```python
from build123d import *

# Parameters (mm, degrees)
SKETCH_1_W                   = 60
SKETCH_1_H                   = 60
EXTRUDE_1_DEPTH              = 4
HOLE_WIZARD_M3_1_D           = 3.4
HOLE_WIZARD_M3_1_CSINK_D     = 6.6
HOLE_WIZARD_M3_1_CSINK_ANGLE = 90
HOLE_WIZARD_M4_1_AT_2_COUNT  = 2
HOLE_WIZARD_M4_1_AT_2_PITCH  = 19
HOLE_WIZARD_M4_1_AT_3_COUNT  = 2
HOLE_WIZARD_M4_1_AT_3_PITCH  = 38
HOLE_WIZARD_1_D              = 3
SKETCH_9_W                   = 12
SKETCH_9_H                   = 19
SKETCH_9_R                   = 1.5
EXTRUDE_3_DEPTH              = 4
CHAMFER_1_SIZE               = 0.5
SKETCH_10_W                  = 72
SKETCH_10_H                  = 4
EXTRUDE_4_DEPTH              = 20


with BuildPart() as part:
    # 草图1 → 凸台-拉伸1 (new body)
    with BuildSketch(Plane(origin=(0, 0, 0), x_dir=(1, 0, 0), z_dir=(0, 1, 0))):
        Rectangle(SKETCH_1_W, SKETCH_1_H)
    extrude(amount=EXTRUDE_1_DEPTH)

    # M3 十字槽沉头木螺钉的锥形沉头孔1 (through all)
    with Locations(Plane(origin=(0, 4, 0), x_dir=(1, 0, 0), z_dir=(0, 1, 0))):
        with Locations((-10, 10), (10, 10), (10, -10), (-10, -10)):
            CounterSinkHole(HOLE_WIZARD_M3_1_D / 2, HOLE_WIZARD_M3_1_CSINK_D / 2, counter_sink_angle=HOLE_WIZARD_M3_1_CSINK_ANGLE)

    # 草图5 → M4 十字槽沉头木螺钉的锥形沉头孔1 (revolve, cut)
    with BuildSketch(Plane(origin=(-19, 0, 0), x_dir=(0, 0, -1), z_dir=(1, 0, 0))):
        Polygon((0, 0), (0, 4), (2.25, 4), (2.25, 2.05), (4.3, 0), align=None)
    hole_wizard_m4_1 = revolve(axis=Axis((-19, -6.35, 0), (0, 1, 0)), mode=Mode.SUBTRACT)

    # M4 十字槽沉头木螺钉的锥形沉头孔1 at 2: M4 十字槽沉头木螺钉的锥形沉头孔1 ×2
    with Locations(*[(i * HOLE_WIZARD_M4_1_AT_2_PITCH, 0, 0) for i in range(1, HOLE_WIZARD_M4_1_AT_2_COUNT)]):
        add(hole_wizard_m4_1, mode=Mode.SUBTRACT)

    # M4 十字槽沉头木螺钉的锥形沉头孔1 at 3: M4 十字槽沉头木螺钉的锥形沉头孔1 ×2
    with Locations(*[(i * HOLE_WIZARD_M4_1_AT_3_PITCH, 0, 0) for i in range(1, HOLE_WIZARD_M4_1_AT_3_COUNT)]):
        add(hole_wizard_m4_1, mode=Mode.SUBTRACT)

    # 孔1 (through all)
    with Locations(Plane(origin=(0, 4, 0), x_dir=(1, 0, 0), z_dir=(0, 1, 0))):
        with Locations((25, 25), (25, -25), (0, -25), (-25, -25), (-25, 25), (0, 25)):
            Hole(HOLE_WIZARD_1_D / 2)

    # 草图9 → 凸台-拉伸3 (add)
    with BuildSketch(Plane(origin=(0, 4, 0), x_dir=(1, 0, 0), z_dir=(0, 1, 0))):
        with Locations((36, -20.5)):
            Rectangle(SKETCH_9_W, SKETCH_9_H)
        with Locations(Location((39, -17, 0), (0, 0, 270))):
            Circle(SKETCH_9_R, mode=Mode.SUBTRACT)
    extrude_3 = extrude(amount=-EXTRUDE_3_DEPTH)

    # 倒角1
    chamfer_1_edges = [part.edges().sort_by_distance(p)[0] for p in [
        (-30, 2, 30),
    ]]
    chamfer(chamfer_1_edges, length=CHAMFER_1_SIZE)

    # 镜向1: 凸台-拉伸3 across plane
    add(extrude_3.mirror(Plane.XY))

    # 草图10 → 凸台-拉伸4 (add)
    with BuildSketch(Plane(origin=(0, 0, -30), x_dir=(-1, 0, 0), z_dir=(0, 0, -1))):
        with Locations((-6, 2)):
            Rectangle(SKETCH_10_W, SKETCH_10_H)
    extrude(amount=EXTRUDE_4_DEPTH)


solid = part.part
```
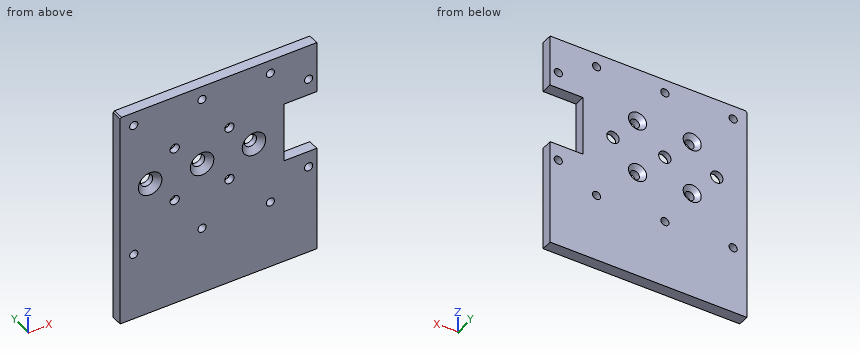
Input: part model. Units: mm. Frame: model coordinates. Coordinates: 2 decimals unless noted, no trailing zeros. Loops run counter-clockwise (first coordinate to the right, second up) from the corner with the lowest first, then second, coordinate; pieces in that order, holes last. Notation, with made-up numbers: (-6.75, 80) -> (41.25, 80) arc R18 ccw to (41.25, 107) -> close; hole circle Ø11 at (-25.75, -8). An arc over 180 degrees is marked (long way). Use a Markdown table: item, result.
1) Cut plane A-A (x = 39). Return the cut outline in (y, z), then the cut area to 3 significant figures.
Results found:
| item | result |
|---|---|
| outline | (0, -50) -> (4, -50) -> (4, -18.5) -> (0, -18.5) -> close; (0, -15.5) -> (4, -15.5) -> (4, -11) -> (0, -11) -> close; (0, 11) -> (4, 11) -> (4, 15.5) -> (0, 15.5) -> close; (0, 18.5) -> (4, 18.5) -> (4, 30) -> (0, 30) -> close |
| area | 208 mm2 |
2) Contact query for flat-ended pins moving along their axis: pin 1 (2 mm diameter, centred on y = 2.5, z = -1.5, fed in from +X); pin 2 (2.5 mm diameter, centred on x = 10, z = 10, fed in from +Y) (3 decimals); pin 3 (4.5 mm diameter, centred on x = -10, z = -10, fed in from +Y). Output: stop coordinate, or through.
Results found:
| item | result |
|---|---|
| pin 1 | stops at x = 30 |
| pin 2 | passes through |
| pin 3 | stops at y = 2.95 |
3) Material intervals for line 1 along X through (y, z) = (2.7, 0); line 2 along X through (y, z) = (2.45, -25); line 3 along X through (y, z) = (1.3, -10), sorted ascending. Write a range as from..to.
Results found:
| item | result |
|---|---|
| line 1 | x = -30..-21.25, -16.75..-2.25, 2.25..16.75, 21.25..30 |
| line 2 | x = -30..-26.5, -23.5..-1.5, 1.5..23.5, 26.5..42 |
| line 3 | x = -30..-11.7, -8.3..8.3, 11.7..30 |
4) Cut plane B-B (z = 0). Return the cut outline in (x, y).
Results found:
| item | result |
|---|---|
| outline | (-30, 0) -> (-23.3, 0) -> (-21.25, 2.05) -> (-21.25, 4) -> (-30, 4) -> close; (-16.75, 2.05) -> (-14.7, 0) -> (-4.3, 0) -> (-2.25, 2.05) -> (-2.25, 4) -> (-16.75, 4) -> close; (2.25, 2.05) -> (4.3, 0) -> (14.7, 0) -> (16.75, 2.05) -> (16.75, 4) -> (2.25, 4) -> close; (21.25, 2.05) -> (23.3, 0) -> (30, 0) -> (30, 4) -> (21.25, 4) -> close |
5) Cut plane D-D (x = 10). Return the cut outline in (y, z), then the cut area to 3 significant figures.
Results found:
| item | result |
|---|---|
| outline | (0, -50) -> (4, -50) -> (4, -13.3) -> (2.4, -11.7) -> (0, -11.7) -> close; (0, -8.3) -> (2.4, -8.3) -> (4, -6.7) -> (4, 6.7) -> (2.4, 8.3) -> (0, 8.3) -> close; (0, 11.7) -> (2.4, 11.7) -> (4, 13.3) -> (4, 30) -> (0, 30) -> close |
| area | 288 mm2 |
6) Cut plane C-C (y = 3.2). Give the number of separate pieces and of enclosed holes in the cut face, then the cut area to 3 significant figures.
Results found:
| item | result |
|---|---|
| separate pieces | 1 |
| enclosed holes | 15 |
| area | 5,310 mm2 |
